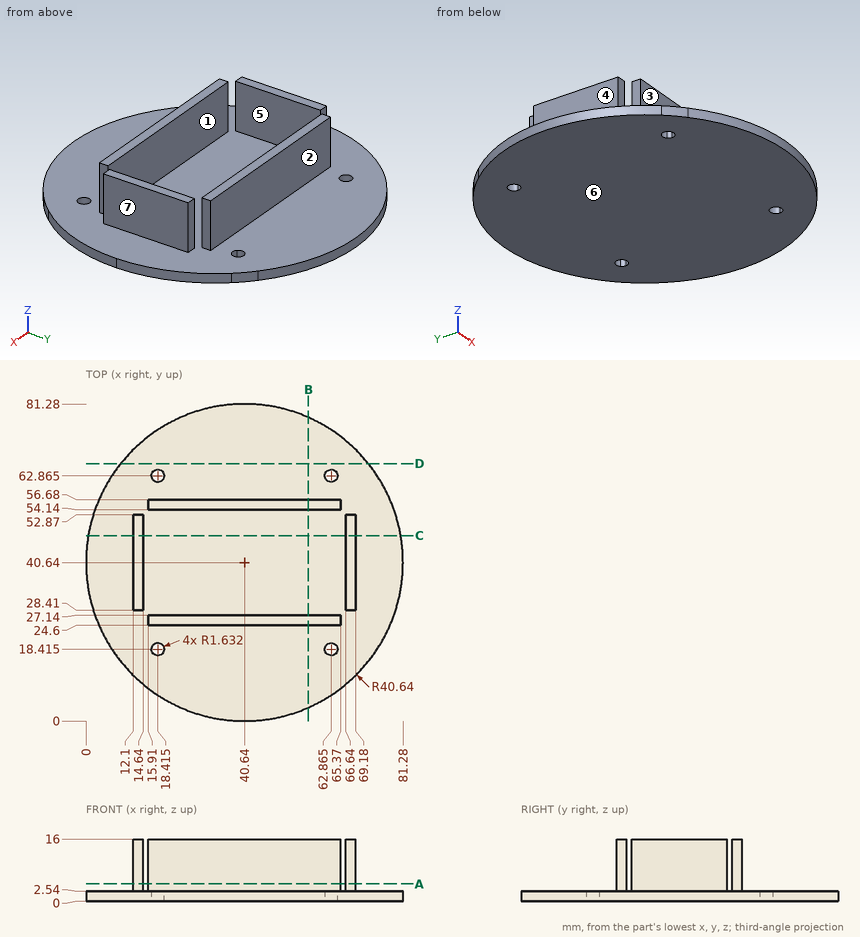
Design review of the part shown in the three views and the two pictorial views. Dimensions are in mm from the part's minimum x, y and z. A direction names the side the tool comes from. Give positions to 0.01 mm unless a question says otherwise; leave off trailing zeros. Order: outer loops, then holes, each group sorted by start corner. A loop starts at its lowest first (then second) coordinate and runs counter-clockwise, first axis right, second up. Notation, with made-up numbers: M 12,15.5 L 41,15.5 A29 ccw 41,39.5 Z; hole C -34.75,71.25 d10. An arc over 180 degrees is marked long. Answer in a Markdown table with one row per item. Add a question column.
(1) Consider section C-C on y = 47.5. State the section outline as (x, z) points, and give its area (3 significant figures).
(2) Wall thickness on probe 1 along Y at (x, z) = (33, 5); probe 2 along X at (y, z) = (51, 12.25); probe 3 along Z at (x, y) = (49, 15): over which ranges is each line inside the solid? List them lowest first. Write a range as [from, to].
(3) For pin 1 (1.3 mm diameter, centred on x = 68, z = 9.5, fed in from +Y); pin 2 (1 mm diameter, centred on x = 49.5, y = 33.5, fed in from +Z); pin 3 (1.5 mm diameter, centred on y = 30, z = 4, fed in from +X); pin 4 (12 mm diameter, centred on x = 38.5, y = 20, fed in from -Z), all flat-tipped, find the tip position at first contact; note any pin that passes through.
(4) Consider section A-A on z = 4.5. State the section outline as (x, y) points.
(5) Consider section D-D on y = 66. State the section outline as (x, z) points, and give its area (3 significant figures).
(6) Mouldability with a two-part tool opening along Y and no side actions: class the marked faces 1, 2 and 3 as +Y half, -Y half, draft (parallel to the pull), parting line (faces both ways), or undercut.
(7) For the marked faces 4, 5, 6 and 7, list the 3-axis set-ups (+Z, -Z, +X, -X, +Y, -Y) from which the entire face can be reached by the end or side of a thin tool; tool diameter is ignored.
(8) Consider section B-B on x = 57. State the section outline as (y, z) points.
Evaluation:
| question | item | result |
|---|---|---|
| 1 | outline | M 0.58,0 L 80.7,0 L 80.7,2.54 L 69.18,2.54 L 69.18,16 L 66.64,16 L 66.64,2.54 L 14.64,2.54 L 14.64,16 L 12.1,16 L 12.1,2.54 L 0.58,2.54 Z |
| 1 | area | 272 mm^2 |
| 2 | probe 1 | y = [24.6, 27.14], [54.14, 56.68] |
| 2 | probe 2 | x = [12.1, 14.64], [66.64, 69.18] |
| 2 | probe 3 | z = [0, 2.54] |
| 3 | pin 1 | stops at y = 52.87 |
| 3 | pin 2 | stops at z = 2.54 |
| 3 | pin 3 | stops at x = 69.18 |
| 3 | pin 4 | stops at z = 0 |
| 4 | outline | M 12.1,28.41 L 14.64,28.41 L 14.64,52.87 L 12.1,52.87 Z; M 15.91,24.6 L 65.37,24.6 L 65.37,27.14 L 15.91,27.14 Z; M 15.91,54.14 L 65.37,54.14 L 65.37,56.68 L 15.91,56.68 Z; M 66.64,28.41 L 69.18,28.41 L 69.18,52.87 L 66.64,52.87 Z |
| 5 | outline | M 8.88,0 L 72.4,0 L 72.4,2.54 L 8.88,2.54 Z |
| 5 | area | 161 mm^2 |
| 6 | face 1 | undercut |
| 6 | face 2 | +Y half |
| 6 | face 3 | -Y half |
| 7 | face 4 | +Z, -X, +Y, -Y |
| 7 | face 5 | +Z, +Y, -Y |
| 7 | face 6 | -Z, +X, -X, +Y, -Y |
| 7 | face 7 | +Z, +X, +Y, -Y |
| 8 | outline | M 3.44,0 L 77.84,0 L 77.84,2.54 L 56.68,2.54 L 56.68,16 L 54.14,16 L 54.14,2.54 L 27.14,2.54 L 27.14,16 L 24.6,16 L 24.6,2.54 L 3.44,2.54 Z |
